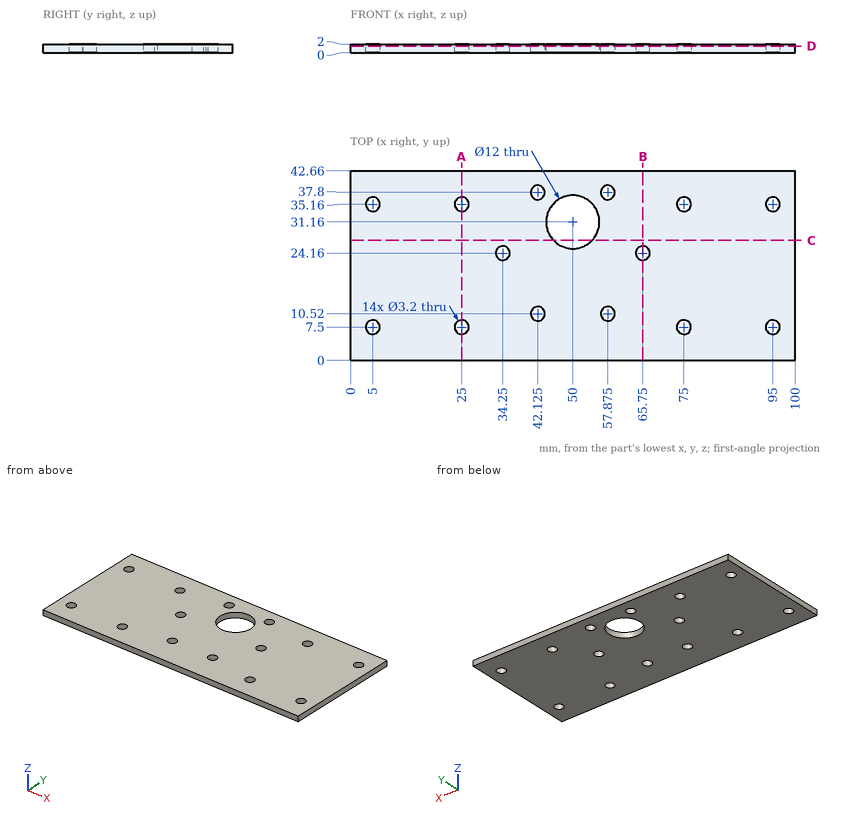
Geometry: see drawing. Coordinates: mm, zero at the bounding-box minimum. Coordinates: 2 decimals unless noted, no trailing zeros. Order: outer loops, then holes, each group sorted by start corner. A loop starts at its lowest first (then second) coordinate and runs counter-clockwise, first axis right, second up. Notation, with made-up numbers: M -39,35.25 L 20,35.25 A18 ccw 20,58.25 Z; hole C 73.25,29.25 d1. An arc over 180 degrees is marked long. Answer as CSV lines item,"result".
1. Section A-A (x = 25). Return the cut outline in (y, z), then the cut area to 3 significant figures.
Reported:
outline,"M 0,0 L 5.9,0 L 5.9,2 L 0,2 Z; M 9.1,0 L 33.56,0 L 33.56,2 L 9.1,2 Z; M 36.76,0 L 42.66,0 L 42.66,2 L 36.76,2 Z"
area,"72.5 mm2"
2. Section D-D (z = 1.5). State how many separate pieces and enclosed holes the cut face has, then the cut area to 3 significant figures.
Reported:
separate pieces,"1"
enclosed holes,"15"
area,"4,040 mm2"
3. Section B-B (x = 65.75). Return the cut outline in (y, z).
Reported:
outline,"M 0,0 L 22.56,0 L 22.56,2 L 0,2 Z; M 25.76,0 L 42.66,0 L 42.66,2 L 25.76,2 Z"
4. First-contact query: P1, Ø3, axis at x = 5, y = 7.5, coming from the +Z side. Flat tip, straight axial feed; report the tip coordinate or a pass-through.
Reported:
P1,"through"
5. Section C-C (y = 27). Return the cut outline in (x, z), then the cut area to 3 significant figures.
Reported:
outline,"M 0,0 L 45.68,0 L 45.68,2 L 0,2 Z; M 54.32,0 L 100,0 L 100,2 L 54.32,2 Z"
area,"183 mm2"
6. Material intervals for line 1 (Y direction, x = 75, z = 1.05); line 2 (Y direction, x = 50, z = 1.65); line 3 (X direction, y = 35, z = 1.05), sorted ascending. Write a range as from..to.
Reported:
line 1,"0..5.9, 9.1..33.56, 36.76..42.66"
line 2,"0..25.16, 37.16..42.66"
line 3,"0..3.41, 6.59..23.41, 26.59..45.39, 54.61..73.41, 76.59..93.41, 96.59..100"
